Could you check a few things on this model? Use its own coordinates, in mm. Give positions to 0.01 mm unless a question says otherwise; leave off trailing zeros. Loops run counter-clockwise (first coordinate to the right, second up) from the corner with the lowest first, then second, coordinate; pieces in that order, holes last. Notation, with made-up numbers: M -23,69.25 L 21,69.25 A26 cw 21,84.25 Z; hole C -14,10 d7. An arc over 180 degrees is marked long. Answer in a Markdown table with one row per item. Add a question column.
1. If we section it at A-A on z = 0: List the corners of the cut face in (x, y) for me.
2. If we section it at B-B on z = -20.5: List the corners of the cut face in (x, y) for me.
3. I need wall thicknesses on line 1 along Y through (x, z) = (-38.5, -11); line 2 along Y through (x, z) = (57.5, -1); line 3 along Z through (x, y) = (-148, -147). Which ranges of each line are inside material? Lowest first, please. Write a range as from..to.
4. I'm going to push flat-ended pins straight in: pin 1 Ø2 at (x, y) = (77.5, -25.5) entering from -Z; pin 2 Ø21 at (y, z) = (5.5, 5.5) entering from -X; pin 3 Ø6 at (x, z) = (-36.5, 21) entering from -Y. Where does each tip first touch, or does it pass through?
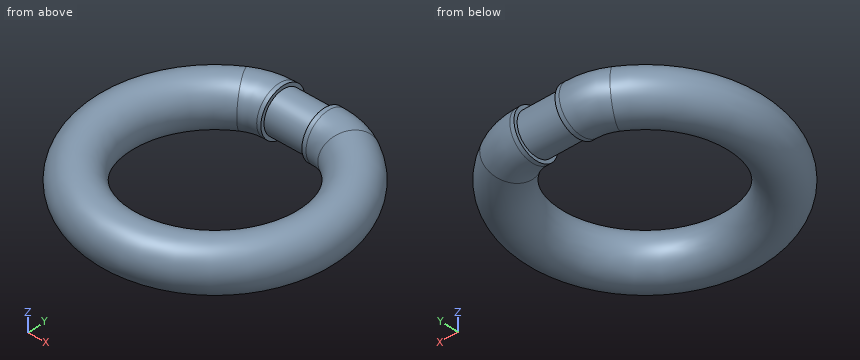
```python
from build123d import *

# Parameters (mm, degrees)
SKETCH_1_W = 60
SKETCH_1_H = 30
SKETCH_3_R = 35


with BuildPart() as part:
    # Эскиз1 → Повернуть1 (revolve)
    with BuildSketch(Plane.XY):
        with Locations((0, 15)):
            Rectangle(SKETCH_1_W, SKETCH_1_H)
    revolve(axis=Axis((-50.256410256, 0, 0), (1, 0, 0)))

    # По траектории1: sweep along a path in Эскиз2
    with BuildLine(Plane.XY) as sweep_1_path:
        Line((-30, 0), (-36.055512755, 0))
        ThreePointArc((-36.055512755, 0), (-57.436412108, -2.910071067), (-77.261813046, -11.428571429))
        ThreePointArc((-77.261813046, -11.428571429), (0, -290), (77.261813046, -11.428571429))
        ThreePointArc((77.261813046, -11.428571429), (57.436412108, -2.910071067), (36.055512755, 0))
        Line((36.055512755, 0), (30, 0))
    # Эскиз3 → По траектории1 (sweep)
    with BuildSketch(Plane.ZY.offset(30)):
        Circle(SKETCH_3_R)
    sweep(path=sweep_1_path.line)


solid = part.part
```
Results:
| question | item | result |
|---|---|---|
| 1 | outline | M -95.29,18.57 A185 ccw long 95.29,18.57 A115 ccw 36.06,35 L 30,35 L 30,30 L -30,30 L -30,35 L -36.06,35 A115 ccw Z; hole M -59.23,-41.43 A115 ccw long 59.23,-41.43 A45 ccw 36.06,-35 L 30,-35 L 30,-30 L -30,-30 L -30,-35 L -36.06,-35 A45 ccw Z |
| 2 | outline | M -91.87,12.89 A178.37 ccw long 91.87,12.89 A108.37 ccw 36.06,28.37 L 30,28.37 L 30,21.9 L -30,21.9 L -30,28.37 L -36.06,28.37 A108.37 ccw Z; hole M -62.65,-35.74 A121.63 ccw long 62.65,-35.74 A51.63 ccw 36.06,-28.37 L 30,-28.37 L 30,-21.9 L -30,-21.9 L -30,-28.37 L -36.06,-28.37 A51.63 ccw Z |
| 3 | line 1 | -319.14..-250.24, -33.29..33.2 |
| 3 | line 2 | -315.82..-239.61, -40.42..32.97 |
| 3 | line 3 | -34.95..34.95 |
| 4 | pin 1 | z = -33.31 |
| 4 | pin 2 | x = -126.04 |
| 4 | pin 3 | y = -316.38 |
